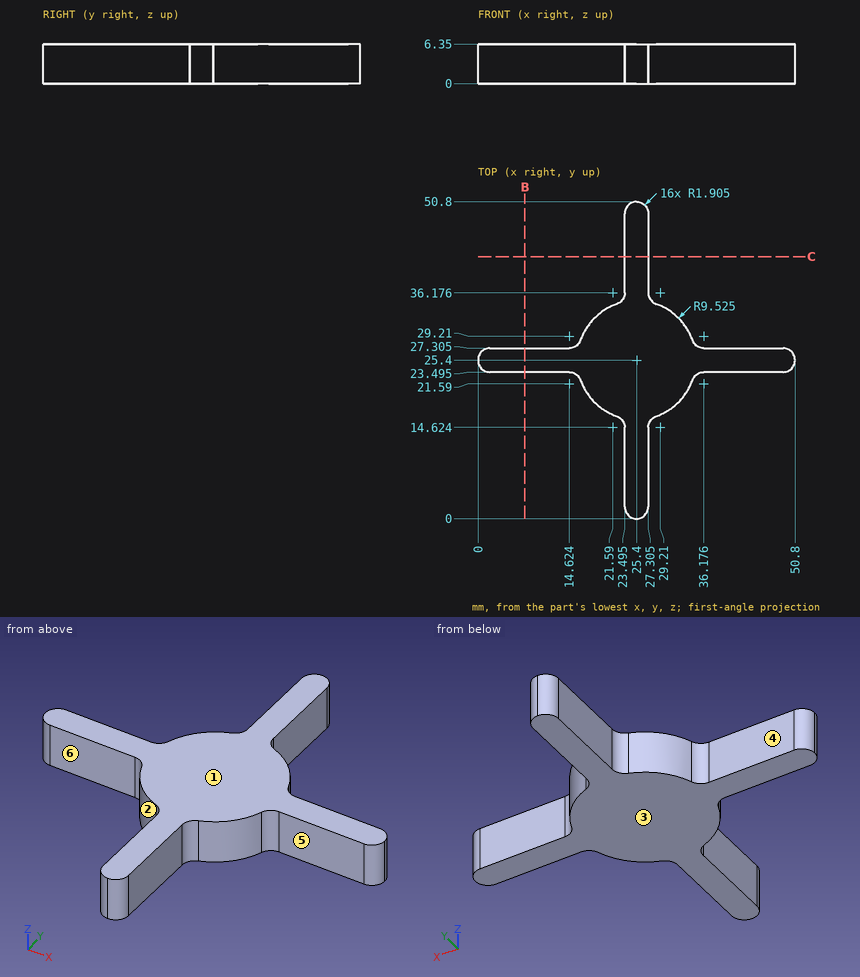
Geometry check sheet. Reference: drawing and pictorial views, mm from the part's lowest x, y, z. A direction names the side the tool comes from. Give positions to 0.01 mm unless a question says otherwise; leave off trailing zeros. Loops run counter-clockwise (first coordinate to the right, second up) from the corner with the lowest first, then second, coordinate; pieces in that order, holes last. Notation, with made-up numbers: (67.5, 54) - (98.5, 54) arc R20 ccw to (98.5, 87) - close; hole circle Ø11 at (34, 40). An arc over 180 degrees is marked (long way). One line per question, with ' | ' between items. Start each with the question number.
1. Cross-section at B-B, the plane x = 7.5. Enter the section's corners in (y, z) (3 decimals).
2. Gauge pin test, flat ends, axial feed: pin 1 Ø3 at (x, z) = (44, 3) entering from +Y (3 decimals); pin 2 Ø2 at (y, z) = (45.5, 4.5) entering from +X (3 decimals); pin 3 Ø2 at (y, z) = (31.5, 1) entering from -X (1 decimal). Record the tip position at first contact, or that the pin passes through.
3. Draft check along Z on the marked faces 1, 2 and 3. Enter one of: released by +Z, released by -Z, zero draft, split by the parting line, or undercut.
4. Set-up check for the marked faces 4, 5 and 6: record each of +Z, -Z, +X, -X, +Y, -Y from which the full face is reachable in a straight line by a thin tool's end or side.
5. Material ranges on line 1 along Y through (x, z) = (39, 5.5) (3 decimals); line 2 along X through (y, z) = (22.5, 0.75), recorded low to high. Write a range as [from, to].
Check result:
1) outline: (23.495, 0) - (27.305, 0) - (27.305, 6.35) - (23.495, 6.35) - close
2) pin 1: stops at y = 27.305 | pin 2: stops at x = 27.305 | pin 3: stops at x = 17.4
3) face 1: released by +Z | face 2: zero draft | face 3: released by -Z
4) face 4: +Z, -Z, -X, +Y | face 5: +Z, -Z, +X, -Y | face 6: +Z, -Z, -X, -Y
5) line 1: y = [23.495, 27.305] | line 2: x = [16.3, 34.5]
